Could you check a few things on this drawing? It's one solid part, dimensions in mm from its lowest x, y, z. A direction names the side the tool comes from. Give positions to 0.01 mm unless a question says otherwise; leave off trailing zeros. Write each loop counter-clockwise with the first axis right and the second up, starting at its lowest first coordinate (ties: lowest second). Pieces come first, ordered by that corner, then holes.
1. Thinking about a two-plate mould opening in X: for the marked faces 1, 2 and 3, which applies, pulls with the +X half, pulls with the -X half, needs draft (parallel to the pull), parting line crosses it, or undercut?
2. I'm going to push flat-ended pins straight in: pin 1 (8 mm diameter, centred on x = 2, y = 9.5, fed in from -Z); pin 2 (1.5 mm diameter, centred on x = 2, z = 0.5, fed in from +Y). Where does each tip first touch, or does it pass through?
3. Suppose I cut it at C-C (z = 0.4). Please give me the cut outline in (x, y), and give its area (3 significant figures).
4. Suppose I cut it at D-D (x = 11.75). Please give me the cut outline in (y, z).
5. If I drill on probe 1 along Y at (x, z) = (7.5, 3.4); probe 2 along Z at (x, y) = (3.25, 11); probe 3 along X at (y, z) = (8.5, 1.9), over which ranges is the centre line in solid material (lowest first)?
6. On a 3-axis mill with a long thin cutter (end or side, diameter ignored), from which of +Z, -Z, +X, -X, +Y, -Y can I reach the whole of each face in a straight line? I mean the marked faces 4 and 5. Say none if no direction works.
7. Suppose I cut it at A-A (y = 7.5). Please give me the cut outline in (x, z).
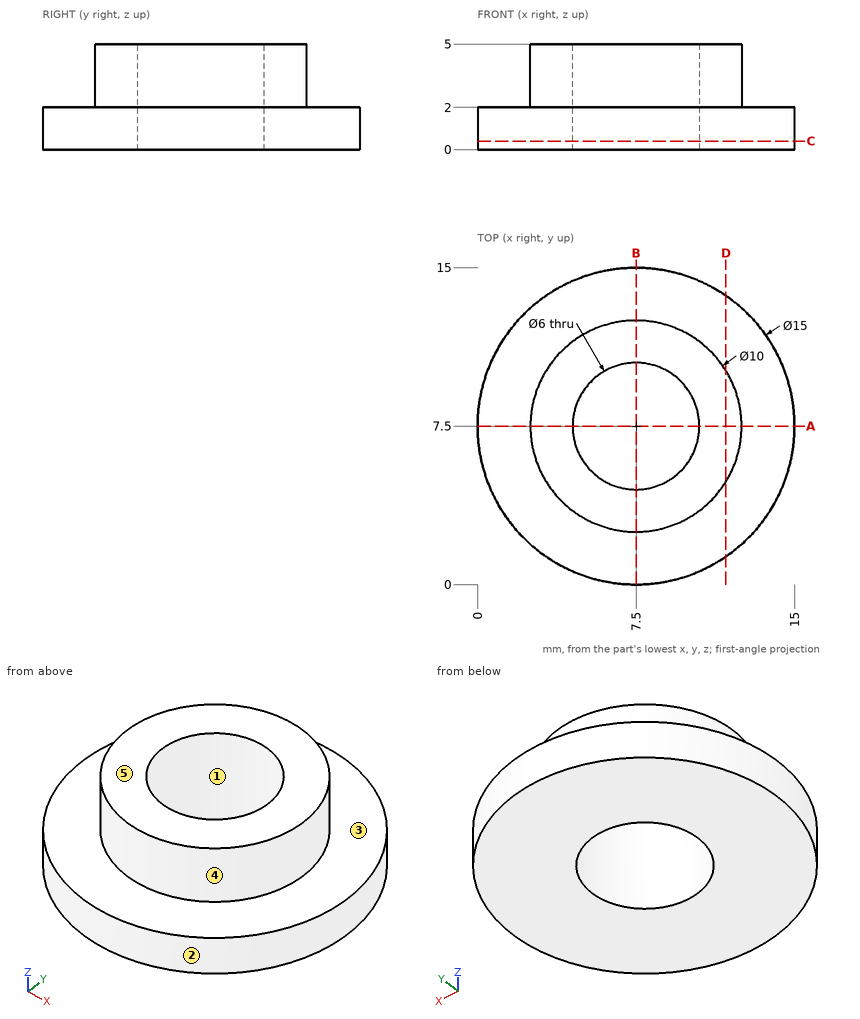
Checks:
1. face 1: undercut
1. face 2: parting line crosses it
1. face 3: needs draft
2. pin 1: stops at z = 0
2. pin 2: stops at y = 13.3
3. outline: circle Ø15 at (7.5, 7.5); hole circle Ø6 at (7.5, 7.5)
3. area: 148 mm2
4. outline: (1.32, 0) - (13.68, 0) - (13.68, 2) - (10.13, 2) - (10.13, 5) - (4.87, 5) - (4.87, 2) - (1.32, 2) - close
5. probe 1: y = 2.5 to 4.5, 10.5 to 12.5
5. probe 2: z = 0 to 2
5. probe 3: x = 0.07 to 4.67, 10.33 to 14.93
6. face 4: +Z
6. face 5: +Z, +X, -X, +Y, -Y
7. outline: (0, 0) - (4.5, 0) - (4.5, 5) - (2.5, 5) - (2.5, 2) - (0, 2) - close; (10.5, 0) - (15, 0) - (15, 2) - (12.5, 2) - (12.5, 5) - (10.5, 5) - close
